from build123d import *

# Parameters (mm, degrees)
BOSS_EXTRUDE1_DEPTH  = 2.6
M4_CLEARANCE_HOLE1_D = 4.8


with BuildPart() as part:
    # Sketch1 → Boss-Extrude1 (new body)
    with BuildSketch(Plane.XY):
        with BuildLine():
            Line((-35.68229717, 9.947502865), (-56.506516782, 46.269686426))
            ThreePointArc((-56.506516782, 46.269686426), (-55.303300859, 55.303300859), (-46.269686426, 56.506516782))
            Line((-46.269686426, 56.506516782), (-9.947502865, 35.68229717))
            ThreePointArc((-9.947502865, 35.68229717), (0, 33.033008589), (9.947502865, 35.68229717))
            Line((9.947502865, 35.68229717), (46.269686426, 56.506516782))
            ThreePointArc((46.269686426, 56.506516782), (55.303300859, 55.303300859), (56.506516782, 46.269686426))
            Line((56.506516782, 46.269686426), (35.68229717, 9.947502865))
            ThreePointArc((35.68229717, 9.947502865), (33.033008589, 0), (35.68229717, -9.947502865))
            Line((35.68229717, -9.947502865), (56.506516782, -46.269686426))
            ThreePointArc((56.506516782, -46.269686426), (55.303300859, -55.303300859), (46.269686426, -56.506516782))
            Line((46.269686426, -56.506516782), (9.947502865, -35.68229717))
            ThreePointArc((9.947502865, -35.68229717), (0, -33.033008589), (-9.947502865, -35.68229717))
            Line((-9.947502865, -35.68229717), (-46.269686426, -56.506516782))
            ThreePointArc((-46.269686426, -56.506516782), (-55.303300859, -55.303300859), (-56.506516782, -46.269686426))
            Line((-56.506516782, -46.269686426), (-35.68229717, -9.947502865))
            ThreePointArc((-35.68229717, -9.947502865), (-33.033008589, 0), (-35.68229717, 9.947502865))
        make_face()
    extrude(amount=BOSS_EXTRUDE1_DEPTH)

    # M4 Clearance Hole1 (through all)
    with Locations(Plane(origin=(0, 0, 0), x_dir=(1, 0, 0), z_dir=(0, 0, -1))):
        with Locations((-50, -50), (-37.5, -37.5), (37.5, -37.5), (50, -50), (50, 50), (37.5, 37.5), (-37.5, 37.5), (-50, 50)):
            Hole(M4_CLEARANCE_HOLE1_D / 2)


solid = part.part
Can you work these out from the model? Positions are in its coordinate system, mm. A direction names the side the tool comes from. Give positions to 0.01 mm unless a question says otherwise; leave off trailing zeros. Order: outer loops, then holes, each group sorted by start corner. A loop starts at its lowest first (then second) coordinate and runs counter-clockwise, first axis right, second up. Notation, with made-up numbers: M 74.25,25 L 92.25,25 A13 cw 92.25,36 Z; hole C -18,33 d6. An arc over 180 degrees is marked long. Use one line per item in the form item = value. Start each with the question number.
Item 1: If we section it at D-D (x = 18.5): Write out the boundary of the cut face in (y, z), then the cut area to 3 significant figures.
Item 2: If we section it at B-B (x = -50): Write out the boundary of the cut face in (y, z), then the cut area to 3 significant figures.
Item 3: We'd pull the mould along X, two halves only. Please class faces 1 (the flat face through (1, 1, 0)), 2 (the cylindrical face through (-33.034, -0.146, 1.282)), 3 (the cylindrical face through (51.905, -48.54, 1.318)), 4 (the flat face through (45.949, -27.854, 1.282)): +X half, -X half, draft (parallel to the pull), parting line (faces both ways), or undercut.
Item 4: If I drill on line 1 along Y through (x, z) = (-50, 0.95); line 2 along Y through (x, z) = (39, 0.25); line 3 along X through (y, z) = (-37.5, 1.2), over which ranges is the centre line in solid material (lowest first)?
Item 5: If we section it at A-A (y = -43.5): Write out the boundary of the cut face in (x, z), then the cut area to 3 significant figures.
Item 6: For faces 5 (the cylindrical face through (-55.205, -55.399, 1.282)), 6 (the flat face through (28.36, -46.24, 1.28)), 7 (the flat face through (46.24, 28.36, 1.28)), 8 (the flat face through (-28.36, 46.24, 1.28)), which set-ups out of +Z, -Z, +X, -X, +Y, -Y let a thin tool reach every point of the face, with its end or its side?
Item 7: If we section it at C-C (y = 37.5): Write out the boundary of the cut face in (x, z), then the cut area to 3 significant figures.
Outcome:
q1.outline = M -40.59,0 L 40.59,0 L 40.59,2.6 L -40.59,2.6 Z
q1.area = 211 mm2
q2.outline = M -57.5,0 L -52.4,0 L -52.4,2.6 L -57.5,2.6 Z; M -47.6,0 L -34.92,0 L -34.92,2.6 L -47.6,2.6 Z; M 34.92,0 L 47.6,0 L 47.6,2.6 L 34.92,2.6 Z; M 52.4,0 L 57.5,0 L 57.5,2.6 L 52.4,2.6 Z
q2.area = 92.5 mm2
q3.face_1 = draft
q3.face_2 = -X half
q3.face_3 = undercut
q3.face_4 = +X half
q4.line_1 = -57.5 to -52.4, -47.6 to -34.92, 34.92 to 47.6, 52.4 to 57.5
q4.line_2 = -52.34 to -39.37, -35.63 to -15.73, 15.73 to 35.63, 39.37 to 52.34
q4.line_3 = -51.48 to -39.9, -35.1 to -13.12, 13.12 to 35.1, 39.9 to 51.48
q5.outline = M -54.92,0 L -23.58,0 L -23.58,2.6 L -54.92,2.6 Z; M 23.58,0 L 54.92,0 L 54.92,2.6 L 23.58,2.6 Z
q5.area = 163 mm2
q6.face_5 = +Z, -Z
q6.face_6 = +Z, -Z, -Y
q6.face_7 = +Z, -Z, +X
q6.face_8 = +Z, -Z, +Y
q7.outline = M -51.48,0 L -39.9,0 L -39.9,2.6 L -51.48,2.6 Z; M -35.1,0 L -13.12,0 L -13.12,2.6 L -35.1,2.6 Z; M 13.12,0 L 35.1,0 L 35.1,2.6 L 13.12,2.6 Z; M 39.9,0 L 51.48,0 L 51.48,2.6 L 39.9,2.6 Z
q7.area = 175 mm2
